Verification items for the finished model (mm, model axes). Give positions to 0.01 mm unless a question says otherwise; leave off trailing zeros. Order: outer loops, then holes, each group sorted by start corner. A loop starts at its lowest first (then second) coordinate and runs counter-clockwise, first axis right, second up. Notation, with made-up numbers: M 87.25,80 L 127.25,80 A20 cw 127.25,94 Z; hole C 13,66.5 d5. An arc over 180 degrees is marked long. Answer as a JSON object with one key per item and string values.
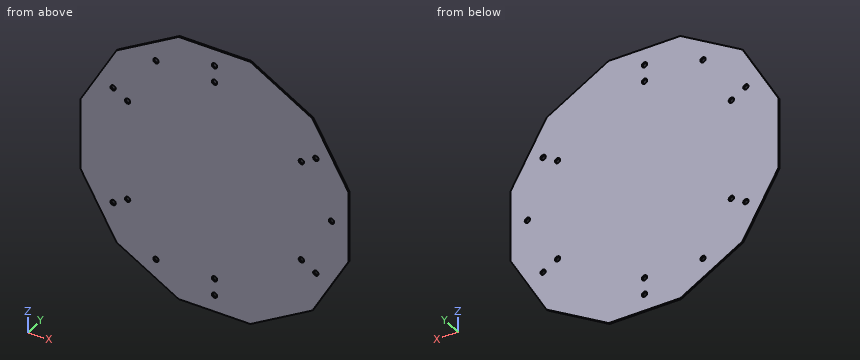
```python
from build123d import *

# Parameters (mm, degrees)
EXTRUDE_2_DEPTH      = 1
SKETCH_9_R           = 1.6
CUT_EXTRUDE_5_DEPTH  = 1
SKETCH_10_R          = 1.6
CUT_EXTRUDE_6_DEPTH  = 1
SKETCH_11_R          = 1.6
CUT_EXTRUDE_7_DEPTH  = 1
SKETCH_12_R          = 1.6
CUT_EXTRUDE_8_DEPTH  = 1
SKETCH_16_R          = 1.6
CUT_EXTRUDE_9_DEPTH  = 1
SKETCH_17_R          = 1.6
CUT_EXTRUDE_10_DEPTH = 1
SKETCH_18_R          = 1.6
CUT_EXTRUDE_11_DEPTH = 1
SKETCH_19_R          = 1.6
CUT_EXTRUDE_12_DEPTH = 1
SKETCH_20_R          = 1.6
CUT_EXTRUDE_13_DEPTH = 1
SKETCH_21_R          = 1.6
CUT_EXTRUDE_14_DEPTH = 1
SKETCH_22_R          = 1.6
CUT_EXTRUDE_15_DEPTH = 1
SKETCH_23_R          = 1.6
CUT_EXTRUDE_16_DEPTH = 1
CUT_EXTRUDE_17_REACH = 3
SKETCH_24_R          = 1.6
CUT_EXTRUDE_18_REACH = 3
SKETCH_25_R          = 1.6
CUT_EXTRUDE_19_REACH = 3
SKETCH_26_R          = 1.6


with BuildPart() as part:
    # ｽｹｯﾁ8 → ﾎﾞｽ - 押し出し2 (new body)
    with BuildSketch(Plane(origin=(0, 0, 0), x_dir=(1, 0, 0), z_dir=(0, 1, 0))):
        Polygon((-80, -21.435935394), (-58.564064606, -58.564064606), (-21.435935394, -80), (21.435935394, -80), (58.564064606, -58.564064606), (80, -21.435935394), (80, 21.435935394), (58.564064606, 58.564064606), (21.435935394, 80), (-21.435935394, 80), (-58.564064606, 58.564064606), (-80, 21.435935394), align=None)
    extrude(amount=EXTRUDE_2_DEPTH)

    # ｽｹｯﾁ9 → ｶｯﾄ - 押し出し5 (cut)
    with BuildSketch(Plane(origin=(0, 1, 0), x_dir=(1, 0, 0), z_dir=(0, 1, 0))):
        with Locations((-60.621778265, 35)):
            Circle(SKETCH_9_R)
    extrude(amount=-CUT_EXTRUDE_5_DEPTH, mode=Mode.SUBTRACT)

    # ｽｹｯﾁ10 → ｶｯﾄ - 押し出し6 (cut)
    with BuildSketch(Plane(origin=(0, 1, 0), x_dir=(1, 0, 0), z_dir=(0, 1, 0))):
        with Locations((-51.961524227, 30)):
            Circle(SKETCH_10_R)
    extrude(amount=-CUT_EXTRUDE_6_DEPTH, mode=Mode.SUBTRACT)

    # ｽｹｯﾁ11 → ｶｯﾄ - 押し出し7 (cut)
    with BuildSketch(Plane(origin=(0, 1, 0), x_dir=(1, 0, 0), z_dir=(0, 1, 0))):
        with Locations((60.621778265, -35)):
            Circle(SKETCH_11_R)
    extrude(amount=-CUT_EXTRUDE_7_DEPTH, mode=Mode.SUBTRACT)

    # ｽｹｯﾁ12 → ｶｯﾄ - 押し出し8 (cut)
    with BuildSketch(Plane(origin=(0, 1, 0), x_dir=(1, 0, 0), z_dir=(0, 1, 0))):
        with Locations((51.961524227, -30)):
            Circle(SKETCH_12_R)
    extrude(amount=-CUT_EXTRUDE_8_DEPTH, mode=Mode.SUBTRACT)

    # ｽｹｯﾁ16 → ｶｯﾄ - 押し出し9 (cut)
    with BuildSketch(Plane(origin=(0, 1, 0), x_dir=(1, 0, 0), z_dir=(0, 1, 0))):
        with Locations((60.621778265, 35)):
            Circle(SKETCH_16_R)
    extrude(amount=-CUT_EXTRUDE_9_DEPTH, mode=Mode.SUBTRACT)

    # ｽｹｯﾁ17 → ｶｯﾄ - 押し出し10 (cut)
    with BuildSketch(Plane(origin=(0, 1, 0), x_dir=(1, 0, 0), z_dir=(0, 1, 0))):
        with Locations((51.961524227, 30)):
            Circle(SKETCH_17_R)
    extrude(amount=-CUT_EXTRUDE_10_DEPTH, mode=Mode.SUBTRACT)

    # ｽｹｯﾁ18 → ｶｯﾄ - 押し出し11 (cut)
    with BuildSketch(Plane(origin=(0, 1, 0), x_dir=(1, 0, 0), z_dir=(0, 1, 0))):
        with Locations((-60.621778265, -35)):
            Circle(SKETCH_18_R)
    extrude(amount=-CUT_EXTRUDE_11_DEPTH, mode=Mode.SUBTRACT)

    # ｽｹｯﾁ19 → ｶｯﾄ - 押し出し12 (cut)
    with BuildSketch(Plane(origin=(0, 1, 0), x_dir=(1, 0, 0), z_dir=(0, 1, 0))):
        with Locations((-51.961524227, -30)):
            Circle(SKETCH_19_R)
    extrude(amount=-CUT_EXTRUDE_12_DEPTH, mode=Mode.SUBTRACT)

    # ｽｹｯﾁ20 → ｶｯﾄ - 押し出し13 (cut)
    with BuildSketch(Plane(origin=(0, 1, 0), x_dir=(1, 0, 0), z_dir=(0, 1, 0))):
        with Locations((0, 70)):
            Circle(SKETCH_20_R)
    extrude(amount=-CUT_EXTRUDE_13_DEPTH, mode=Mode.SUBTRACT)

    # ｽｹｯﾁ21 → ｶｯﾄ - 押し出し14 (cut)
    with BuildSketch(Plane(origin=(0, 1, 0), x_dir=(1, 0, 0), z_dir=(0, 1, 0))):
        with Locations((0, 60)):
            Circle(SKETCH_21_R)
    extrude(amount=-CUT_EXTRUDE_14_DEPTH, mode=Mode.SUBTRACT)

    # ｽｹｯﾁ22 → ｶｯﾄ - 押し出し15 (cut)
    with BuildSketch(Plane(origin=(0, 1, 0), x_dir=(1, 0, 0), z_dir=(0, 1, 0))):
        with Locations((0, -70)):
            Circle(SKETCH_22_R)
    extrude(amount=-CUT_EXTRUDE_15_DEPTH, mode=Mode.SUBTRACT)

    # ｽｹｯﾁ23 → ｶｯﾄ - 押し出し16 (cut)
    with BuildSketch(Plane(origin=(0, 1, 0), x_dir=(1, 0, 0), z_dir=(0, 1, 0))):
        with Locations((0, -60)):
            Circle(SKETCH_23_R)
    extrude(amount=-CUT_EXTRUDE_16_DEPTH, mode=Mode.SUBTRACT)

    # ｽｹｯﾁ24 → ｶｯﾄ - 押し出し17 (cut, up to next)
    with BuildSketch(Plane(origin=(0, 1, 0), x_dir=(1, 0, 0), z_dir=(0, 1, 0)), mode=Mode.PRIVATE) as cut_extrude_17_sk1:
        with Locations((-35, 60.621778265)):
            Circle(SKETCH_24_R)
    cut_extrude_17_tool1 = extrude(cut_extrude_17_sk1.sketch, amount=-CUT_EXTRUDE_17_REACH, mode=Mode.PRIVATE) & part.part
    add(cut_extrude_17_tool1.solids().sort_by_distance((-35, 1, -60.621778))[0], mode=Mode.SUBTRACT)

    # ｽｹｯﾁ25 → ｶｯﾄ - 押し出し18 (cut, up to next)
    with BuildSketch(Plane(origin=(0, 1, 0), x_dir=(1, 0, 0), z_dir=(0, 1, 0)), mode=Mode.PRIVATE) as cut_extrude_18_sk1:
        with Locations((-35, -60.621778265)):
            Circle(SKETCH_25_R)
    cut_extrude_18_tool1 = extrude(cut_extrude_18_sk1.sketch, amount=-CUT_EXTRUDE_18_REACH, mode=Mode.PRIVATE) & part.part
    add(cut_extrude_18_tool1.solids().sort_by_distance((-35, 1, 60.621778))[0], mode=Mode.SUBTRACT)

    # ｽｹｯﾁ26 → ｶｯﾄ - 押し出し19 (cut, up to next)
    with BuildSketch(Plane(origin=(0, 1, 0), x_dir=(1, 0, 0), z_dir=(0, 1, 0)), mode=Mode.PRIVATE) as cut_extrude_19_sk1:
        with Locations((70, 0)):
            Circle(SKETCH_26_R)
    cut_extrude_19_tool1 = extrude(cut_extrude_19_sk1.sketch, amount=-CUT_EXTRUDE_19_REACH, mode=Mode.PRIVATE) & part.part
    add(cut_extrude_19_tool1.solids().sort_by_distance((70, 1, 0))[0], mode=Mode.SUBTRACT)


solid = part.part
```
Q1. Material ranges on L1, parallel to Z at x = 0, y = 0.2; L2, parallel to Z at x = -35.5, y = 0.35; L3, parallel to X at y = 0.7, z = -61, recorded low to high.
Resolved:
{"L1": "z = -80 to -71.6, -68.4 to -61.6, -58.4 to 58.4, 61.6 to 68.4, 71.6 to 80", "L2": "z = -71.88 to -62.14, -59.1 to 59.1, 62.14 to 71.88", "L3": "x = -54.34 to -36.55, -33.45 to -1.25, 1.25 to 54.34"}
Q2. Section check B-B on z = -50.5. Record the cut outline in (x, y), then the cut area to 3 significant figures.
Resolved:
{"outline": "M -63.22,0 L 63.22,0 L 63.22,1 L -63.22,1 Z", "area": "126 mm²"}
Q3. Section check A-A on y = 0.45. Count the separate pieces of the cut face and the enclosed holes in it, then the cut area to 3 significant figures.
Resolved:
{"separate pieces": "1", "enclosed holes": "15", "area": "20,500 mm²"}
Q4. Section check C-C on x = -28.5. Record the cut outline in (y, z), then the cut area to 3 significant figures.
Resolved:
{"outline": "M 0,-75.92 L 1,-75.92 L 1,75.92 L 0,75.92 Z", "area": "152 mm²"}
